Geometry check sheet. Reference: drawing and pictorial views, mm from the part's lowest x, y, z. A direction names the side the tool comes from. Round coordinates to 2 decimals unless told otherwise and drop trailing zeros. Loops run counter-clockwise (first coordinate to the right, second up) from the corner with the lowest first, then second, coordinate; pieces in that order, holes last. Notation, with made-up numbers: (-32.75, -40) - (-15.75, -40) arc R24 cw to (-15.75, -3) - close; hole circle Ø10 at (40.25, -16). An arc over 180 degrees is marked (long way). Put each result on its own line as item: value. Start each with the question number.
Item 1: Section check C-C, the plane x = 20. Record the cut outline in (y, z).
Item 2: Gauge pin test, flat end, axial feed: pin 1 Ø4 at (x, y) = (9.5, 34.75) entering from -Z. Record the tip position at first contact, or that the pin passes through.
Item 3: Section check A-A, the plane z = 27. Record the cut outline in (x, y), and give its area (3 significant figures).
Item 4: Material ranges on line 1 along Y through (x, z) = (44.5, 52.15); line 2 along Z through (x, y) = (27, 4); line 3 along X through (y, z) = (1, 45), recorded low to high.
Item 5: Section check B-B, the plane y = 12. Record the cut outline in (x, z).
Item 6: Section check D-D, the plane y = 7.25. Give the number of separate pieces and of enclosed holes in the cut face, and give its area (3 significant figures).
Item 7: Draft check along Z on the marked faces 3, 4 and 5. Enter one of: pulls with the +Z half, pulls with the -Z half, needs draft (parallel to the pull), parting line crosses it, or undercut.
Item 8: Tool access check on the marked faces 1 and 2. Record the directions out of +Z, -Z, +X, -X, +Y, -Y that give a thin tool (end or side, any length) a straight path to the whole face; none if there is none.
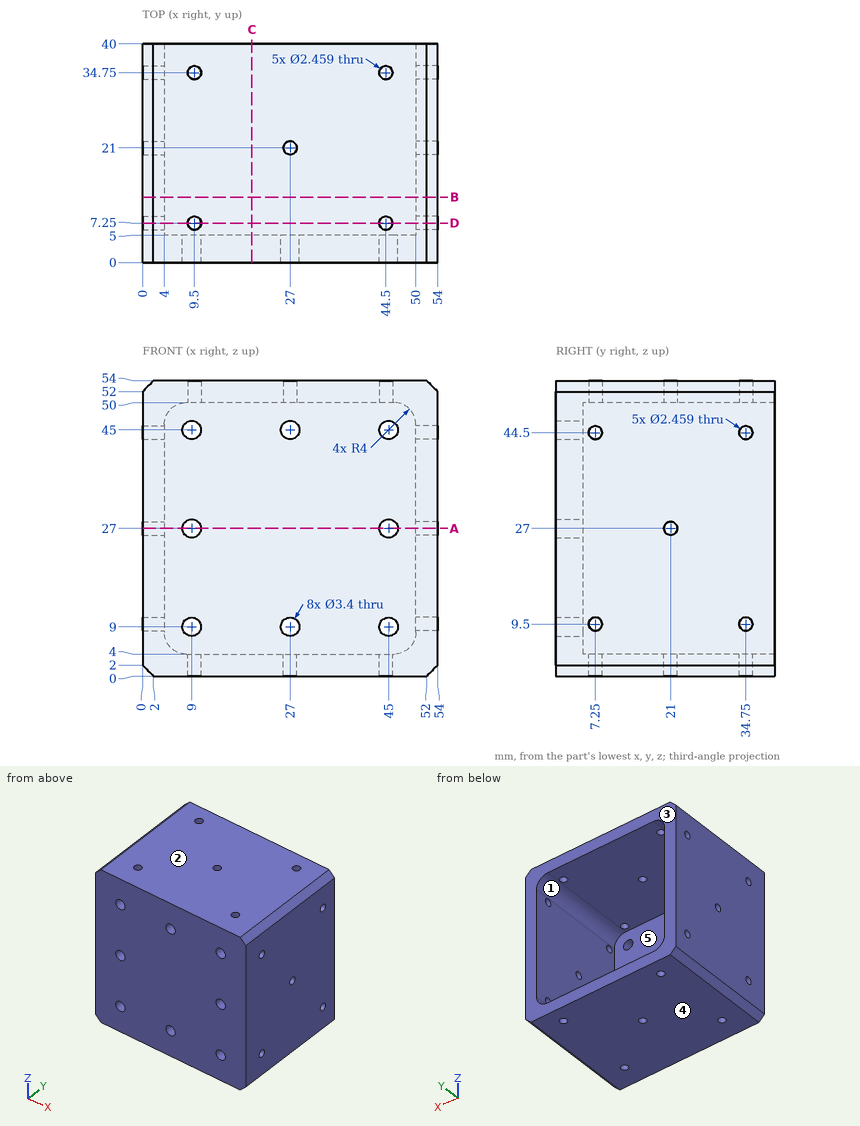
Check result:
1. outline: (0, 0) - (40, 0) - (40, 4) - (5, 4) - (5, 50) - (40, 50) - (40, 54) - (0, 54) - close
2. pin 1: z = 0
3. outline: (0, 0) - (7.3, 0) - (7.3, 5) - (4, 5) - (4, 19.77) - (0, 19.77) - close; (0, 22.23) - (4, 22.23) - (4, 40) - (0, 40) - close; (10.7, 0) - (43.3, 0) - (43.3, 5) - (10.7, 5) - close; (46.7, 0) - (54, 0) - (54, 19.77) - (50, 19.77) - (50, 5) - (46.7, 5) - close; (50, 22.23) - (54, 22.23) - (54, 40) - (50, 40) - close
3. area: 496 mm²
4. line 1: 0 to 6.02, 8.48 to 33.52, 35.98 to 40
4. line 2: 0 to 7.3, 10.7 to 43.3, 46.7 to 54
4. line 3: 0 to 7.3, 10.7 to 25.3, 28.7 to 43.3, 46.7 to 54
5. outline: (0, 2) - (2, 0) - (52, 0) - (54, 2) - (54, 52) - (52, 54) - (2, 54) - (0, 52) - close; hole (4, 8) arc R4 ccw to (8, 4) - (46, 4) arc R4 ccw to (50, 8) - (50, 46) arc R4 ccw to (46, 50) - (8, 50) arc R4 ccw to (4, 46) - close
6. separate pieces: 8
6. enclosed holes: 0
6. area: 727 mm²
7. face 3: needs draft
7. face 4: pulls with the -Z half
7. face 5: undercut
8. face 1: +Y
8. face 2: +Z, +X, -X, +Y, -Y
